```python
from build123d import *

# Parameters (mm, degrees)
CUT_EXTRUDE2_START      = -8
CUT_EXTRUDE2_DEPTH      = 10
CUT_EXTRUDE3_REACH      = 51.487
CUT_EXTRUDE3_END_RADIUS = 3.5
SKETCH3_R               = 1.5
SKETCH4_R               = 1.5
CUT_EXTRUDE5_DEPTH      = 10
CUT_EXTRUDE5_DRAFT      = -15


with BuildPart() as part:
    # Sketch1 → Revolve1 (revolve)
    with BuildSketch(Plane.XY):
        Polygon((3.5, 0), (6, 0), (6, 21), (7.5, 21), (7.5, 28), (10, 28), (10, 45), (3.5, 45), align=None)
    revolve(axis=Axis((0, -1000, 0), (0, 1, 0)))

    # Sketch2 → Cut-Extrude2 (cut)
    with BuildSketch(Plane(origin=(0, 0, 0), x_dir=(0, 0, -1), z_dir=(1, 0, 0)).offset(CUT_EXTRUDE2_START)):
        with BuildLine():
            Line((2, 40), (2, 33))
            ThreePointArc((2, 33), (0, 31), (-2, 33))
            Line((-2, 33), (-2, 40))
            ThreePointArc((-2, 40), (0, 42), (2, 40))
        make_face()
    extrude(amount=-CUT_EXTRUDE2_DEPTH, mode=Mode.SUBTRACT)

    # Cut-Extrude3: up to this cylinder (the profile starts outside it)
    cut_extrude3_end = Plane(origin=(0, 33, 0), z_dir=(0, -1, 0)) * Cylinder(CUT_EXTRUDE3_END_RADIUS, 110.974, mode=Mode.PRIVATE)
    # Sketch3 → Cut-Extrude3 (cut, up to the surface)
    with BuildSketch(Plane.ZY.offset(8), mode=Mode.PRIVATE) as cut_extrude3_sk1:
        with Locations((0, 33)):
            Circle(SKETCH3_R)
    cut_extrude3_tool1 = extrude(cut_extrude3_sk1.sketch, amount=-CUT_EXTRUDE3_REACH, mode=Mode.PRIVATE) - cut_extrude3_end
    add(cut_extrude3_tool1.solids().sort_by_distance((-8, 33, 0))[0], mode=Mode.SUBTRACT)


with BuildPart() as cut_extrude5_tool:
    # Sketch4 → Cut-Extrude5 (with draft: the straight prism first)
    with BuildSketch(Plane(origin=(0, 0, 0), x_dir=(0, 0, -1), z_dir=(1, 0, 0))):
        with Locations(Location((0, 33, 0), (0, 0, 180))):
            Circle(SKETCH4_R)
    extrude(amount=CUT_EXTRUDE5_DEPTH)
    # Cut-Extrude5: the draft: its side faces are tilted about the plane it starts from
    cut_extrude5_sides = [cut_extrude5_tool.faces().sort_by_distance(p)[0] for p in [
        (5, 33, -1.5),
    ]]
    draft(cut_extrude5_sides, Plane(origin=(0, 0, 0), x_dir=(0, 0, -1), z_dir=(1, 0, 0)), CUT_EXTRUDE5_DRAFT)


with BuildPart() as part_1:
    add(part.part)

    # Cut-Extrude5: cut by cut_extrude5_tool
    add(cut_extrude5_tool.part, mode=Mode.SUBTRACT)


solid = part_1.part
```
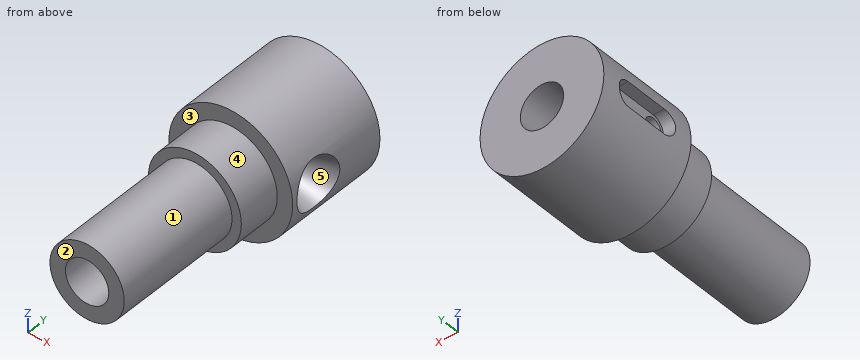
The model under review builds one solid part; all positions refer to its coordinate system, in mm. Face numbers are marked on the shaded views. A direction names the side the tool comes from. Give positions to 0.01 mm unless a question says otherwise; leave off trailing zeros. Write each loop counter-clockwise with the first axis right and the second up, starting at its lowest first coordinate (ties: lowest second). Pieces come first, ordered by that corner, then holes.
(1) Consider section D-D, the plane z = 0. Give the boundary of the cut face in (x, y).
(2) Consider section C-C, the plane x = -7. Give the boundary of the cut face in (y, z).
(3) For P1, Ø2, axis at y = 29, z = -5.5, coming from the +X side; P2, Ø1.4, axis at x = -9.5, y = 38, coming from the +Z side; P3, Ø10, axis at y = 5.5, z = -3.5, coming from the -X side, all flat-tipped, find the tip position at first contact; note any pin that passes through.
(4) Consider section A-A, the plane x = 0. Give the boundary of the cut face in (y, z), and give its area (3 significant figures).
(5) The part is to be moulded in two halves that separate along Y. For the marked faces 3, 4 and 5, say which applies: released by +Y, released by -Y, zero draft, split by the parting line, or undercut.
(6) Consider section B-B, the plane y = 39. Give the boundary of the cut face in (x, z).
(7) Tool access review of the marked faces 1 and 2: name each direction out of +Z, -Z, +X, -X, +Y, -Y from which nothing blocks a thin tool from reaching the whole face with its end or side.
(8) To check wall thickness, follow L1, parallel to Y at x = -4.5, z = 0; L2, parallel to Y at x = -7, z = 0; L3, parallel to Z at x = 0, y = 33. State the ranges of each line that lie inside material, in increasing order.
Returned:
1. outline: (-10, 28) - (-7.5, 28) - (-7.5, 21) - (-6, 21) - (-6, 0) - (-3.5, 0) - (-3.5, 31.5) - (-8, 31.5) - (-8, 31) - (-10, 31) - close; (-10, 42) - (-8, 42) - (-8, 34.5) - (-3.5, 34.5) - (-3.5, 45) - (-10, 45) - close; (3.5, 0) - (6, 0) - (6, 21) - (7.5, 21) - (7.5, 28) - (10, 28) - (10, 28.82) - (3.5, 30.56) - close; (3.5, 35.44) - (10, 37.18) - (10, 45) - (3.5, 45) - close
2. outline: (21, -2.69) - (28, -2.69) - (28, -7.14) - (45, -7.14) - (45, 7.14) - (28, 7.14) - (28, 2.69) - (21, 2.69) - close; hole circle Ø3 at (33, 0)
3. P1: stops at x = 8.93
3. P2: stops at z = 4.75
3. P3: stops at x = -6
4. outline: (0, -6) - (21, -6) - (21, -7.5) - (28, -7.5) - (28, -10) - (45, -10) - (45, -3.5) - (0, -3.5) - close; (0, 3.5) - (45, 3.5) - (45, 10) - (28, 10) - (28, 7.5) - (21, 7.5) - (21, 6) - (0, 6) - close
4. area: 382 mm2
5. face 3: released by -Y
5. face 4: zero draft
5. face 5: undercut
6. outline: (-9.8, -2) arc R10 ccw (long way) to (-9.8, 2) - (-8, 2) - (-8, -2) - close; hole circle Ø7 at (0, 0)
7. face 1: -Y
7. face 2: +Z, -Z, +X, -X, -Y
8. L1: y = 0 to 31.5, 34.5 to 45
8. L2: y = 21 to 31.5, 34.5 to 45
8. L3: z = -10 to -3.5, 3.5 to 10
